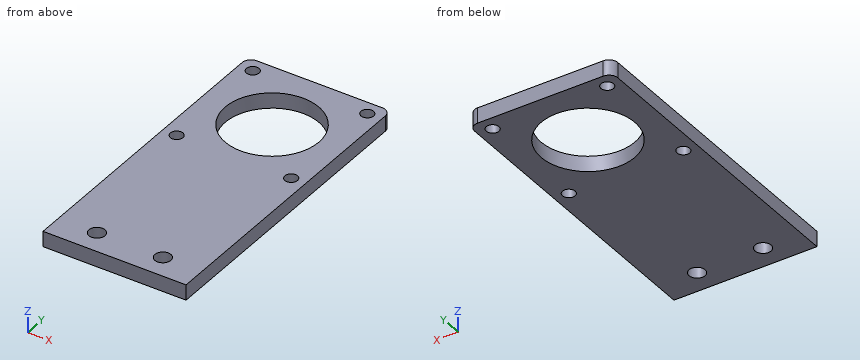
Autodesk Inventor part; units mm, degrees
ref_plane "YZ Plane" through (0, 0, 0) normal (1, 0, 0) x (0, 1, 0)
ref_plane "XZ Plane" through (0, 0, 0) normal (0, 1, 0) x (-1, 0, 0)
ref_plane "XY Plane" through (0, 0, 0) normal (0, 0, 1) x (1, 0, 0)
sketch "Sketch1" plane through (0, 0, 0) normal (0, 0, 1) x (1, 0, 0)
  line L0 (0, 0) -> (58.8772, 0)
  line L1 (58.8772, 0) -> (58.8772, 127)
  line L2 (58.8772, 127) -> (0, 127)
  line L3 (0, 127) -> (0, 0)
  dimension "d0" = 58.8772
  dimension "d1" = 127
extrude "Extrusion1" add sketch "Sketch1" along normal blind 6.35
sketch "Sketch2" plane through (0, 0, 6.35) normal (0, 0, 1) x (1, 0, 0)
  circle A0 centre (29.4386, 97.5614) radius 19.304
  line L0 (58.8772, 127) -> (0, 127)
  line L1 (0, 127) -> (0, 0)
  line L2 (58.8772, 0) -> (58.8772, 127)
  line L3 (29.4386, 127) -> (29.4386, 0)
  line L4 (0, 0) -> (58.8772, 0)
  dimension "d4" = 38.608
  dimension "d5" = 29.4386
extrude "Extrusion2" cut sketch "Sketch2" against normal blind 6.35 contours A0 L3 | L3 A0
sketch "Sketch3" plane through (0, 0, 6.35) normal (0, 0, 1) x (1, 0, 0)
  circle A0 centre (5.8166, 121.1834) radius 2.6035
  line L0 (58.8772, 127) -> (0, 127)
  line L1 (0, 127) -> (0, 0)
  circle A1 centre (5.8166, 74.041) radius 2.6035
  circle A2 centre (52.959, 121.1834) radius 2.6035
  circle A3 centre (52.959, 74.041) radius 2.6035
  dimension "d10" = 5.207
  dimension "d11" = 5.8166
  dimension "d12" = 5.8166
  dimension "d15" = 47.1424
  dimension "d18" = 47.1424
extrude "Extrusion3" cut sketch "Sketch3" against normal blind 6.35
fillet "Fillet1" radius 3.6068 2 edges at (0, 127, 3.175) (58.8772, 127, 3.175)
sketch "Sketch4" plane through (0, 0, 6.35) normal (0, 0, 1) x (1, 0, 0)
  circle A0 centre (15.875, 9.525) radius 3.302
  circle A1 centre (43.0022, 9.525) radius 3.302
  line L0 (0, 0) -> (58.8772, 0)
  line L1 (58.8772, 0) -> (58.8772, 123.3932)
  line L2 (0, 123.3932) -> (0, 0)
  dimension "d24" = 6.604
  dimension "d25" = 6.604
  dimension "d26" = 9.525
  dimension "d27" = 9.525
  dimension "d28" = 15.875
  dimension "d29" = 15.875
extrude "Extrusion4" cut sketch "Sketch4" against normal blind 25.4
properties part number "Motor Support" material "Aluminum 6061"
The listing builds one solid part. Answer for the finished solid, in the listing's coordinates (mm). Give positions to 0.01 mm unless a question says otherwise; leave off trailing zeros. Loops run counter-clockwise (first coordinate to the right, second up) from the corner with the lowest first, then second, coordinate; pieces in that order, holes last. Notation, with made-up numbers: (35, 82) - (79, 82) arc R23 cw to (79, 90) - close; hole circle Ø1 at (55, 66). An arc over 180 degrees is marked (long way). Answer as a JSON object with one key per item and string values.
1. Find the intervals of material crossed by L1, parallel to Y at x = 6, z = 2.5; L2, parallel to X at y = 121, z = 5.5; L3, parallel to Y at x = 41, z = 5, in increasing order. Write a range as [from, to].
Determined:
{"L1": "[0, 71.44], [76.64, 118.59], [123.78, 127]", "L2": "[0, 3.22], [8.41, 50.36], [55.56, 58.88]", "L3": "[0, 6.9], [12.15, 82.1], [113.02, 127]"}
2. A flat-ended cylindrical pin translates along its axis: pin 1 Ø4 at (x, y) = (43, 9.52) entering from +Z. Find the tip coordinate at first contact, or state that the pin passes through.
Determined:
{"pin 1": "through"}
3. A cutting plane is placed at D-D (x = 36). Write down the section's boundary in (y, z), then the cut area to 3 significant figures.
Determined:
{"outline": "(0, 0) - (79.41, 0) - (79.41, 6.35) - (0, 6.35) - close; (115.72, 0) - (127, 0) - (127, 6.35) - (115.72, 6.35) - close", "area": "576 mm²"}
4. A cutting plane is placed at B-B (x = 17.5). Write down the section's boundary in (y, z), then the cut area to 3 significant figures.
Determined:
{"outline": "(0, 0) - (6.65, 0) - (6.65, 6.35) - (0, 6.35) - close; (12.4, 0) - (82.39, 0) - (82.39, 6.35) - (12.4, 6.35) - close; (112.73, 0) - (127, 0) - (127, 6.35) - (112.73, 6.35) - close", "area": "577 mm²"}
5. A cutting plane is placed at A-A (y = 89). Write down the section's boundary in (x, z), then the cut area to 3 significant figures.
Determined:
{"outline": "(0, 0) - (12.14, 0) - (12.14, 6.35) - (0, 6.35) - close; (46.74, 0) - (58.88, 0) - (58.88, 6.35) - (46.74, 6.35) - close", "area": "154 mm²"}
6. A cutting plane is placed at C-C (z = 4.5). Write down the section's boundary in (x, y) (1 decimal).
Determined:
{"outline": "(0, 0) - (58.9, 0) - (58.9, 123.4) arc R3.6 ccw to (55.3, 127) - (3.6, 127) arc R3.6 ccw to (0, 123.4) - close; hole circle Ø5.2 at (5.8, 74); hole circle Ø5.2 at (5.8, 121.2); hole circle Ø38.6 at (29.4, 97.6); hole circle Ø6.6 at (15.9, 9.5); hole circle Ø6.6 at (43, 9.5); hole circle Ø5.2 at (53, 74); hole circle Ø5.2 at (53, 121.2)"}
